from build123d import *

# Parameters (mm, degrees)
SKETCH1_W           = 116
SKETCH1_H           = 60
SKETCH1_W_2         = 110
SKETCH1_H_2         = 54
BOSS_EXTRUDE1_DEPTH = 24
SKETCH2_W           = 116
SKETCH2_H           = 60
BOSS_EXTRUDE2_DEPTH = 3
CUT_EXTRUDE1_DEPTH  = 12.5
BOSS_EXTRUDE3_DEPTH = 12
SKETCH5_W           = 113.4
SKETCH5_H           = 57.4
SKETCH5_W_2         = 110
SKETCH5_H_2         = 54
CUT_EXTRUDE2_DEPTH  = 5.5
CUT_EXTRUDE3_REACH  = 77.802
SKETCH6_W           = 6
SKETCH6_H           = 12
FILLET3_R           = 3


with BuildPart() as part:
    # Sketch1 → Boss-Extrude1 (new body)
    with BuildSketch(Plane(origin=(0, 9.820251789, 0), x_dir=(1, 0, 0), z_dir=(0, 1, 0))):
        Rectangle(SKETCH1_W, SKETCH1_H)
        Rectangle(SKETCH1_W_2, SKETCH1_H_2, mode=Mode.SUBTRACT)
    extrude(amount=BOSS_EXTRUDE1_DEPTH)

    # Sketch2 → Boss-Extrude2 (add)
    with BuildSketch(Plane(origin=(0, 33.820251789, 0), x_dir=(1, 0, 0), z_dir=(0, 1, 0))):
        Rectangle(SKETCH2_W, SKETCH2_H)
    extrude(amount=BOSS_EXTRUDE2_DEPTH)

    # Sketch3 → Cut-Extrude1 (cut, symmetric)
    with BuildSketch(Plane(origin=(0, 0, 0), x_dir=(0, 0, -1), z_dir=(1, 0, 0))):
        Polygon((28.5, 9.820251789), (28.5, 23.320251789), (30, 24.820251789), (30, 9.820251789), align=None)
    cut_extrude1 = extrude(amount=CUT_EXTRUDE1_DEPTH, both=True, mode=Mode.SUBTRACT)

    # Sketch4 → Boss-Extrude3 (add, symmetric)
    with BuildSketch(Plane(origin=(0, 0, 0), x_dir=(0, 0, -1), z_dir=(1, 0, 0))):
        Polygon((30.1, 7.070251789), (28.5, 7.070251789), (28.5, 6.420251789), (30.5, 4.420251789), (32.5, 6.420251789), (36.5, 4.420251789), (36.5, 9.420251789), (31, 16.420251789), (31, 35.820251789), (30, 36.820251789), (29, 36.820251789), (29, 10.734465351), (30.1, 9.634465351), align=None)
    boss_extrude3 = extrude(amount=BOSS_EXTRUDE3_DEPTH, both=True)

    # Sketch5 → Cut-Extrude2 (cut)
    with BuildSketch(Plane.XZ.offset(-9.820251789)):
        Rectangle(SKETCH5_W, SKETCH5_H)
        Rectangle(SKETCH5_W_2, SKETCH5_H_2, mode=Mode.SUBTRACT)
    extrude(amount=-CUT_EXTRUDE2_DEPTH, mode=Mode.SUBTRACT)

    # Mirror1: Cut-Extrude1, Boss-Extrude3 across plane
    add(cut_extrude1.mirror(Plane.XY), mode=Mode.SUBTRACT)
    add(boss_extrude3.mirror(Plane.XY))

    # Sketch6 → Cut-Extrude3 (cut, up to next)
    with BuildSketch(Plane(origin=(0, 36.820251789, 0), x_dir=(1, 0, 0), z_dir=(0, 1, 0)), mode=Mode.PRIVATE) as cut_extrude3_sk1:
        with Locations((-20, 0)):
            Rectangle(SKETCH6_W, SKETCH6_H)
    cut_extrude3_tool1 = extrude(cut_extrude3_sk1.sketch, amount=-CUT_EXTRUDE3_REACH, mode=Mode.PRIVATE) & part.part
    add(cut_extrude3_tool1.solids().sort_by_distance((-20, 36.820252, 0))[0], mode=Mode.SUBTRACT)

    # Fillet3
    fillet3_edges = [part.edges().sort_by_distance(p)[0] for p in [
        (-23, 35.320251789, 6),
        (-17, 35.320251789, 6),
        (-17, 35.320251789, -6),
        (-23, 35.320251789, -6),
    ]]
    fillet(fillet3_edges, radius=FILLET3_R - 0.0001)  # a hair under: the kernel refuses the full size


solid = part.part
Geometry check sheet. Reference: the model listing, model coordinates, mm. A direction names the side the tool comes from. Give positions to 0.01 mm unless a question says otherwise; leave off trailing zeros. Loops run counter-clockwise (first coordinate to the right, second up) from the corner with the lowest first, then second, coordinate; pieces in that order, holes last. Notation, with made-up numbers: (-15, -4.75) -> (26, -4.75) arc R25 cw to (26, 30.25) -> close; hole circle Ø9 at (24, 46). An arc over 180 degrees is marked (long way). Answer in a Markdown table with one row per item. Add a question column.
1) Gauge pin test, flat ends, axial feed: P1, Ø1.5, axis at x = 3, y = 29.5, coming from the +Z side; P2, Ø6.5, axis at x = -4, y = 16, coming from the -Z side; P3, Ø12, axis at x = -43.5, y = 30.5, coming from the +Z side. Record the tip position at first contact, or that the pin passes through.
2) Draft check along Y on faces 5 (the face through (-17, 35, 0)), 6 (the face through (0.168, 5.434, 34.472)), 7 (the face through (0, 17, -29)). Enter one of: pulls with the +Y half, pulls with the -Y half, needs draft (parallel to the pull), parting line crosses it, or undercut.
3) Material ranges on probe 1 along X at (y, z) = (29.5, 10); probe 2 along Z at (x, y) = (52, 30); probe 3 along Z at (x, y) = (-41, 11), recorded low to high. Write a range as from..to.
4) Cross-section at B-B on x = -34.5. Record the boundary of the cut face in (y, z), and give its area (3 significant figures).
5) Cross-section at D-D on z = -25.5. Record the boundary of the cut face in (x, y).
6) Set-up check for faces 1 (the face through (55, 24, 0)), 2 (the face through (-35, 23, -30)), 3 (the face through (-35, 23, 30)), 4 (the face through (0, 19, -28.5)): record each of +Z, -Z, +X, -X, +Y, -Y from which the full face is reachable in a straight line by a thin tool's end or side.
7) Cross-section at A-A on y = 18. Record the boundary of the cut face in (x, z).
8) Cross-section at C-C on y = 32. Record the boundary of the cut face in (x, z).
Outcome:
| question | item | result |
|---|---|---|
| 1 | P1 | stops at z = 31 |
| 1 | P2 | stops at z = -33.88 |
| 1 | P3 | stops at z = 30 |
| 2 | face 5 | needs draft |
| 2 | face 6 | pulls with the -Y half |
| 2 | face 7 | undercut |
| 3 | probe 1 | x = -58..-55, 55..58 |
| 3 | probe 2 | z = -30..-27, 27..30 |
| 3 | probe 3 | z = -30..-28.7, 28.7..30 |
| 4 | outline | (9.82, -30) -> (36.82, -30) -> (36.82, 30) -> (9.82, 30) -> (9.82, 28.7) -> (15.32, 28.7) -> (15.32, 27) -> (33.82, 27) -> (33.82, -27) -> (15.32, -27) -> (15.32, -28.7) -> (9.82, -28.7) -> close |
| 4 | area | 305 mm^2 |
| 5 | outline | (-58, 9.82) -> (-56.7, 9.82) -> (-56.7, 15.32) -> (-55, 15.32) -> (-55, 33.82) -> (55, 33.82) -> (55, 15.32) -> (56.7, 15.32) -> (56.7, 9.82) -> (58, 9.82) -> (58, 36.82) -> (-58, 36.82) -> close |
| 6 | face 1 | -Y |
| 6 | face 2 | -Z, -X, +Y, -Y |
| 6 | face 3 | +Z, -X, +Y, -Y |
| 6 | face 4 | none |
| 7 | outline | (-58, -30) -> (-12.5, -30) -> (-12.5, -28.5) -> (12.5, -28.5) -> (12.5, -30) -> (58, -30) -> (58, 30) -> (12.5, 30) -> (12.5, 28.5) -> (-12.5, 28.5) -> (-12.5, 30) -> (-58, 30) -> close; (-12, -31) -> (12, -31) -> (12, -29) -> (-12, -29) -> close; (-12, 29) -> (12, 29) -> (12, 31) -> (-12, 31) -> close; hole (-55, -27) -> (55, -27) -> (55, 27) -> (-55, 27) -> close |
| 8 | outline | (-58, -30) -> (-12, -30) -> (-12, -31) -> (12, -31) -> (12, -30) -> (58, -30) -> (58, 30) -> (12, 30) -> (12, 31) -> (-12, 31) -> (-12, 30) -> (-58, 30) -> close; hole (-55, -27) -> (55, -27) -> (55, 27) -> (-55, 27) -> close |
